from build123d import *

# Parameters (mm, degrees)
F0_R     = 14.3129
F1_DEPTH = 25.4


with BuildPart() as f1:
    # F0 (on Front) → F1 (new body)
    with BuildSketch(Plane.XZ):
        with BuildLine():
            Line((-38.447507, 39.146728), (-51.203564, 39.146728))
            Line((-51.203564, 39.146728), (-51.203564, -28.671272))
            Line((-51.203564, -28.671272), (126.596436, -28.671272))
            Line((126.596436, -28.671272), (126.596436, 39.146728))
            Line((126.596436, 39.146728), (117.981013, 39.146728))
            ThreePointArc((117.981013, 39.146728), (116.836108, 38.87406), (115.691204, 39.146728))
            Line((115.691204, 39.146728), (-36.157697, 39.146728))
            ThreePointArc((-36.157697, 39.146728), (-37.302602, 38.87406), (-38.447507, 39.146728))
        make_face()
        with Locations((42.271748, 22.790955)):
            Circle(F0_R, mode=Mode.SUBTRACT)
    extrude(amount=F1_DEPTH)


solid = f1.part
CAD build for the part. Positions are in the model's coordinates, mm. Give positions to 0.01 mm unless a question says otherwise; leave off trailing zeros. Loops run counter-clockwise (first coordinate to the right, second up) from the corner with the lowest first, then second, coordinate; pieces in that order, holes last. Notation, with made-up numbers: M 30.5,28.25 L 89.5,28.25 A11 cw 89.5,44.25 Z; hole C 83,59 d11. An arc over 180 degrees is marked long. One line per question, with ' | ' between items. Start each with the question number.
1. Saw through at C-C on y = -20. Give the cut face in (x, z).
2. Probe L1, parallel to X at y = -2, z = 35; L2, parallel to X at y = -20.75, z = 16.5; L3, parallel to Z at x = 40, y = -11.75. List the from-to ranges inside material, lowest first. Write a range as from..to.
3. Saw through at A-A on x = 47.5. Give the cut face in (y, z).
4. Saw through at B-B on z = 35. Give the cut face in (x, y), plus the area to 3 significant figures.
Result sheet:
1) outline: M -51.2,-28.67 L 126.6,-28.67 L 126.6,39.15 L 117.98,39.15 A2.54 cw 115.69,39.15 L -36.16,39.15 A2.54 cw -38.45,39.15 L -51.2,39.15 Z; hole C 42.27,22.79 d28.63
2) L1: x = -51.2..34.8, 49.74..126.6 | L2: x = -51.2..29.42, 55.13..126.6 | L3: z = -28.67..8.66, 36.92..39.15
3) outline: M -25.4,-28.67 L 0,-28.67 L 0,9.47 L -25.4,9.47 Z; M -25.4,36.11 L 0,36.11 L 0,39.15 L -25.4,39.15 Z
4) outline: M -51.2,-25.4 L 34.8,-25.4 L 34.8,0 L -51.2,0 Z; M 49.74,-25.4 L 126.6,-25.4 L 126.6,0 L 49.74,0 Z | area: 4,140 mm^2
